Work out the finished part from the listing and answer in its coordinate system (mm). A direction names the side the tool comes from. Give positions to 0.01 mm unless a question says otherwise; leave off trailing zeros. Loops run counter-clockwise (first coordinate to the right, second up) from the corner with the lowest first, then second, coordinate; pieces in that order, holes last. Notation, with made-up numbers: (-10, 20.5) - (16, 20.5) arc R17 ccw to (16, 25.5) - close; hole circle Ø4 at (21.5, 40.5). An arc over 180 degrees is marked (long way). One line per item, written item: value.
from build123d import *

# Parameters (mm, degrees)
SKETCH1_R                = 2
SKETCH1_R_2              = 69.5
BOSS_EXTRUDE3_DEPTH      = 1.5
BOSS_EXTRUDE3_DEPTH_BACK = 1.5
SKETCH2_R                = 72.5
SKETCH2_R_2              = 69.5
BOSS_EXTRUDE4_DEPTH      = 40
SKETCH4_R                = 75
SKETCH4_R_2              = 72
BOSS_EXTRUDE6_DEPTH      = 40


with BuildPart() as part:
    # Sketch1 → Boss-Extrude3 (new, two sides)
    with BuildSketch(Plane(origin=(0, 0, 0), x_dir=(1, 0, 0), z_dir=(0, 1, 0))) as boss_extrude3_sk:
        with BuildLine():
            Line((80, 90), (-80, 90))
            ThreePointArc((-80, 90), (-87.071067812, 87.071067812), (-90, 80))
            Line((-90, 80), (-90, -80))
            ThreePointArc((-90, -80), (-87.071067812, -87.071067812), (-80, -90))
            Line((-80, -90), (80, -90))
            ThreePointArc((80, -90), (87.071067812, -87.071067812), (90, -80))
            Line((90, -80), (90, 80))
            ThreePointArc((90, 80), (87.071067812, 87.071067812), (80, 90))
        make_face()
        with Locations(Location((-80, -80, 0), (0, 0, 270))):
            Circle(SKETCH1_R, mode=Mode.SUBTRACT)
        with Locations(Location((80, -80, 0), (0, 0, 270))):
            Circle(SKETCH1_R, mode=Mode.SUBTRACT)
        with Locations(Location((80, 80, 0), (0, 0, 270))):
            Circle(SKETCH1_R, mode=Mode.SUBTRACT)
        with Locations(Location((-80, 80, 0), (0, 0, 270))):
            Circle(SKETCH1_R, mode=Mode.SUBTRACT)
        with Locations(Location((0, 0, 0), (0, 0, 270))):
            Circle(SKETCH1_R_2, mode=Mode.SUBTRACT)
    extrude(amount=BOSS_EXTRUDE3_DEPTH)
    extrude(boss_extrude3_sk.sketch, amount=-BOSS_EXTRUDE3_DEPTH_BACK)

    # Sketch2 → Boss-Extrude4 (add)
    with BuildSketch(Plane(origin=(0, 0, 0), x_dir=(1, 0, 0), z_dir=(0, 1, 0))):
        with Locations(Location((0, 0, 0), (0, 0, 270))):
            Circle(SKETCH2_R)
        with Locations(Location((0, 0, 0), (0, 0, 270))):
            Circle(SKETCH2_R_2, mode=Mode.SUBTRACT)
    extrude(amount=BOSS_EXTRUDE4_DEPTH)

    # Sketch4 → Boss-Extrude6 (add)
    with BuildSketch(Plane(origin=(0, 0, 0), x_dir=(1, 0, 0), z_dir=(0, 1, 0))):
        with Locations(Location((0, 0, 0), (0, 0, 270))):
            Circle(SKETCH4_R)
        with Locations(Location((0, 0, 0), (0, 0, 270))):
            Circle(SKETCH4_R_2, mode=Mode.SUBTRACT)
    extrude(amount=-BOSS_EXTRUDE6_DEPTH)


solid = part.part
1. Section B-B (z = 0) is taken. Write down the section's boundary in (x, y), and give its area (3 significant figures).
Output:
outline: (-90, -1.5) - (-75, -1.5) - (-75, -40) - (-72, -40) - (-72, -1.5) - (-69.5, -1.5) - (-69.5, 40) - (-72.5, 40) - (-72.5, 1.5) - (-90, 1.5) - close; (69.5, -1.5) - (72, -1.5) - (72, -40) - (75, -40) - (75, -1.5) - (90, -1.5) - (90, 1.5) - (72.5, 1.5) - (72.5, 40) - (69.5, 40) - close
area: 585 mm²
2. Section C-C (y = -26.5) is taken. Write down the section's boundary in (x, z).
Output:
outline: circle Ø150 at (0, 0); hole circle Ø144 at (0, 0)
3. Flat-ended cylindrical pins translate along their axes: pin 1 Ø3 at (x, z) = (-80, 80) entering from +Y; pin 2 Ø5 at (y, z) = (10.5, 18.5) entering from -X; pin 3 Ø4.5 at (x, z) = (80, 80) entering from +Y; pin 4 Ø5 at (x, y) = (4, 22) entering from -Z. Find the tip coordinate at first contact, or state that the pin passes through.
Output:
pin 1: passes through
pin 2: stops at x = -70.71
pin 3: stops at y = 1.5
pin 4: stops at z = -72.48
4. Section D-D (y = 21.5) is taken. Write down the section's boundary in (x, z).
Output:
outline: circle Ø145 at (0, 0); hole circle Ø139 at (0, 0)
5. Find the intervals of material crossed by line 1 along X through (y, z) = (0, 80); line 2 along X through (y, z) = (-1, 0); line 3 along X through (y, z) = (-16.5, 0), in increasing order.
Output:
line 1: x = -90 to -82, -78 to 78, 82 to 90
line 2: x = -90 to -69.5, 69.5 to 90
line 3: x = -75 to -72, 72 to 75
6. For faces 4 (the cylindrical face through (-87.15, 0.02, 86.99)), 5 (the cylindrical face through (21.78, 20.48, 69.15)), 6 (the cylindrical face through (21.627, -20.48, 68.675)), determine the directions among +Z, -Z, +X, -X, +Y, -Y from which every point of the face is accessible in a straight line to the end or side of a thin tool.
Output:
face 4: +Z, -X, +Y, -Y
face 5: +Y
face 6: -Y
7. The mould has two halves that part along X. Classify faces 1 (the flat face through (-38, -1.5, -59)), 2 (the flat face through (67, -40, -28)), 3 (the cylindrical face through (-86.99, 0.02, -87.15)): released by +X, released by -X, zero draft, split by the parting line, or undercut.
Output:
face 1: undercut
face 2: zero draft
face 3: released by -X
8. Section A-A (x = 0) is taken. Write down the section's boundary in (y, z), and give its area (3 significant figures).
Output:
outline: (-40, -75) - (-1.5, -75) - (-1.5, -90) - (1.5, -90) - (1.5, -72.5) - (40, -72.5) - (40, -69.5) - (-1.5, -69.5) - (-1.5, -72) - (-40, -72) - close; (-40, 72) - (-1.5, 72) - (-1.5, 69.5) - (40, 69.5) - (40, 72.5) - (1.5, 72.5) - (1.5, 90) - (-1.5, 90) - (-1.5, 75) - (-40, 75) - close
area: 585 mm²
